```python
from build123d import *

# Parameters (mm, degrees)
EXTRUDE_1_DEPTH     = 10
SKETCH_2_R          = 1.55
SKETCH_2_R_2        = 8
CUT_EXTRUDE_1_DEPTH = 10
CUT_EXTRUDE_2_DEPTH = 25
FILLET_1_R          = 1.5
SKETCH_4_R          = 6.5
CUT_EXTRUDE_3_DEPTH = 25
EXTRUDE_START       = -10
EXTRUDE_2_DEPTH     = 10


with BuildPart() as part:
    # 草图1 → 凸台-拉伸1 (new body)
    with BuildSketch(Plane.XY):
        with BuildLine():
            Line((105.880667011, 9.774167654), (1.281264399, 17.453033018))
            ThreePointArc((1.281264399, 17.453033018), (-17.494246359, 0.448714084), (0.384854302, -17.495767693))
            Line((0.384854302, -17.495767693), (105.240374084, -15.189261425))
            ThreePointArc((105.240374084, -15.189261425), (117.461368411, -3.012794561), (105.880667011, 9.774167654))
        make_face()
    extrude(amount=EXTRUDE_1_DEPTH)

    # 草图2 → 切除-拉伸1 (cut)
    with BuildSketch(Plane.XY.offset(10)):
        with Locations((0, 13.5)):
            Circle(SKETCH_2_R)
        with Locations((11.691342951, 6.75)):
            Circle(SKETCH_2_R)
        with Locations((11.691342951, -6.75)):
            Circle(SKETCH_2_R)
        with Locations((0, -13.5)):
            Circle(SKETCH_2_R)
        with Locations((-11.691342951, -6.75)):
            Circle(SKETCH_2_R)
        with Locations((-11.691342951, 6.75)):
            Circle(SKETCH_2_R)
        Circle(SKETCH_2_R_2)
    extrude(amount=-CUT_EXTRUDE_1_DEPTH, mode=Mode.SUBTRACT)

    # 草图3 → 切除-拉伸2 (cut)
    with BuildSketch(Plane.XY.offset(10)):
        Polygon((28.969702276, -12.866019337), (97.16669186, -11.365890548), (78.883612283, -1.217324734), align=None)
        Polygon((26.667415907, 11.578617262), (18.617416428, -10.147636057), (91.362216416, 6.829233896), align=None)
    extrude(amount=-CUT_EXTRUDE_2_DEPTH, mode=Mode.SUBTRACT)

    # 圆角1
    fillet_1_edges = [part.edges().sort_by_distance(p)[0] for p in [
        (26.667415907, 11.578617262, 5),
        (91.362216416, 6.829233896, 5),
        (18.617416428, -10.147636057, 5),
        (28.969702276, -12.866019337, 5),
        (78.883612283, -1.217324734, 5),
        (97.16669186, -11.365890548, 5),
    ]]
    fillet(fillet_1_edges, radius=FILLET_1_R)

    # 草图4 → 切除-拉伸3 (cut)
    with BuildSketch(Plane.XY.offset(10)):
        with Locations((104.965478154, -2.692284502)):
            Circle(SKETCH_4_R)
    extrude(amount=-CUT_EXTRUDE_3_DEPTH, mode=Mode.SUBTRACT)

    # 草图5 → 凸台-拉伸2 (add)
    with BuildSketch(Plane.XY.offset(10).offset(EXTRUDE_START)):
        with BuildLine():
            Line((93.666088337, 10.670865941), (105.880667011, 9.774167654))
            ThreePointArc((105.880667011, 9.774167654), (117.461368411, -3.012794561), (105.240374084, -15.189261425))
            Line((105.240374084, -15.189261425), (92.995887368, -15.458603329))
            ThreePointArc((92.995887368, -15.458603329), (122.459724513, -3.140998585), (93.666088337, 10.670865941))
        make_face()
    extrude(amount=EXTRUDE_2_DEPTH)


solid = part.part
```
Geometry check sheet. Reference: the model listing, model coordinates, mm. A direction names the side the tool comes from. Give positions to 0.01 mm unless a question says otherwise; leave off trailing zeros. Order: outer loops, then holes, each group sorted by start corner. A loop starts at its lowest first (then second) coordinate and runs counter-clockwise, first axis right, second up. Notation, with made-up numbers: (10, -36.75) - (18, -36.75) arc R11 cw to (18, -18.75) - close; hole circle Ø10 at (-34.75, -14.5). An arc over 180 degrees is marked (long way). Answer in a Markdown table with one row per item. Add a question column.
Q1. Mould release check, pull along X, two halves, no side actions. Record for faces 3 (the flat face through (52, -5, 10)), 4 (the cylindrical face through (10.46, -7.69, 5.07)): pulls with the +X half, pulls with the -X half, needs draft (parallel to the pull), parting line crosses it, or undercut.
Q2. Material ranges on probe 1 along Y at (x, z) = (0, 3.75); probe 2 along X at (y, z) = (6, 2.5); probe 3 along Y at (x, z) = (43, 2), recorded low to high. Write a range as from..to.
Q3. Cross-section at C-C, the plane x = 67. Enter the section's corners in (y, z), then the cut area to 3 significant figures.
Q4. Gauge pin test, flat ends, axial feed: pin 1 (3 mm diameter, centred on x = 85, z = 8, fed in from -Y); pin 2 (3 mm diameter, centred on x = -11.69, y = -6.75, fed in from +Z); pin 3 (3 mm diameter, centred on y = -4.5, z = 5, fed in from +X); pin 4 (1.5 mm diameter, centred on y = -12, z = 4, fed in from -X). Record the tip position at first contact, or that the pin passes through.
Q5. Cross-section at B-B, the plane z = 2.75. Count the separate pieces of the cut face and the enclosed holes in it, then the cut area to 3 significant figures.
Q6. Tool access check on faces 1 (the flat face through (48.12, 14.014, 4.93)), 2 (the flat face through (51.13, -2.56, 5.07)). Record the directions out of +Z, -Z, +X, -X, +Y, -Y that give a thin tool (end or side, any length) a straight path to the whole face; none if there is none.
Q7. Cross-section at A-A, the plane x = 110. Enter the section's corners in (y, z).
Check values:
| question | item | result |
|---|---|---|
| 1 | face 3 | needs draft |
| 1 | face 4 | undercut |
| 2 | probe 1 | y = -17.5..-15.05, -11.95..-8, 8..11.95, 15.05..17.5 |
| 2 | probe 2 | x = -16.44..-13.05, -10.33..-5.29, 5.29..10.33, 13.05..24.6, 82.94..120.15 |
| 2 | probe 3 | y = -16.56..-12.51, -9.59..-4.46, 10.38..14.39 |
| 3 | outline | (-16.03, 0) - (-12.03, 0) - (-12.03, 10) - (-16.03, 10) - close; (-3.99, 0) - (1.14, 0) - (1.14, 10) - (-3.99, 10) - close; (8.62, 0) - (12.63, 0) - (12.63, 10) - (8.62, 10) - close |
| 3 | area | 131 mm^2 |
| 4 | pin 1 | stops at y = -15.67 |
| 4 | pin 2 | passes through |
| 4 | pin 3 | stops at x = 122.46 |
| 4 | pin 4 | stops at x = -13.4 |
| 5 | separate pieces | 1 |
| 5 | enclosed holes | 10 |
| 5 | area | 2,770 mm^2 |
| 6 | face 1 | +Z, -Z, +Y |
| 6 | face 2 | +Z, -Z |
| 7 | outline | (-19.45, 0) - (-6.8, 0) - (-6.8, 10) - (-19.45, 10) - close; (1.42, 0) - (14.07, 0) - (14.07, 10) - (1.42, 10) - close |
